Work out the finished part from the listing and answer in its coordinate system (mm). Round coordinates to 2 decimals unless told otherwise and drop trailing zeros. Write each loop counter-clockwise with the first axis right and the second up, starting at its lowest first coordinate (ties: lowest second). Pieces come first, ordered by that corner, then holes. Notation, with made-up numbers: (50.25, 76.5) -> (58.25, 76.5) arc R33 cw to (58.25, 108.5) -> close; hole circle Ø7 at (-17.75, 27.5). An arc over 180 degrees is marked (long way). One line per item, written item: value.
```python
from build123d import *

# Parameters (mm, degrees)
SZKIC1_R                    = 11
DODANIE_WYCI_GNI_CIE1_DEPTH = 5.25
ZAOKR_GLENIE1_R             = 0.2


with BuildPart() as part:
    # Szkic1 → Dodanie-wyciągnięcie1 (new body, symmetric)
    with BuildSketch(Plane(origin=(0, 0, 0), x_dir=(1, 0, 0), z_dir=(0, 1, 0))):
        Circle(SZKIC1_R)
    extrude(amount=DODANIE_WYCI_GNI_CIE1_DEPTH, both=True)

    # Szkic3 → Wycięcie-obrót1 (revolve, cut)
    with BuildSketch(Plane.XY):
        with BuildLine():
            Line((0, -9.52), (0, 9.52))
            ThreePointArc((0, 9.52), (9.52, 0), (0, -9.52))
        make_face()
    revolve(axis=Axis((0, -9.52, 0), (0, 1, 0)), mode=Mode.SUBTRACT)

    # Zaokrąglenie1
    zaokr_glenie1_edges = [part.edges().sort_by_distance(p)[0] for p in [
        (-11, -5.25, 0),
        (-11, 5.25, 0),
    ]]
    fillet(zaokr_glenie1_edges, radius=ZAOKR_GLENIE1_R)


solid = part.part
```
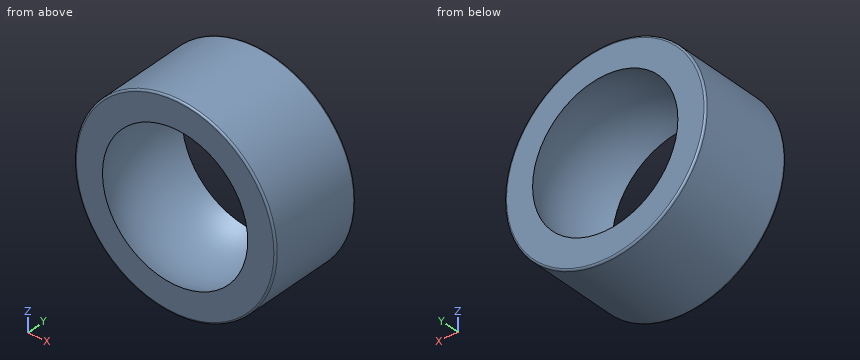
(1) Find section A-A on z = 0. Give the vertices of the cut face in (x, y), plus the area to 3 significant figures.
Reported:
outline: (-11, -5.05) arc R0.2 ccw to (-10.8, -5.25) -> (-7.94, -5.25) arc R9.52 cw to (-7.94, 5.25) -> (-10.8, 5.25) arc R0.2 ccw to (-11, 5.05) -> close; (7.94, -5.25) -> (10.8, -5.25) arc R0.2 ccw to (11, -5.05) -> (11, 5.05) arc R0.2 ccw to (10.8, 5.25) -> (7.94, 5.25) arc R9.52 cw to start
area: 41.7 mm2
(2) Find section D-D on y = -3.5. Give the vertices of the cut face in (x, z).
Reported:
outline: circle Ø22 at (0, 0); hole circle Ø17.71 at (0, 0)
(3) Flat-ended cylindrical pins translate along their axes: pin 1 Ø4 at (y, z) = (3.5, 4.5) entering from -X; pin 2 Ø4 at (y, z) = (-0.5, 4) entering from -X; pin 3 Ø6 at (x, y) = (-5, -3.5) entering from -Z. Find the tip coordinate at first contact, or state that the pin passes through.
Reported:
pin 1: stops at x = -10.71
pin 2: stops at x = -10.82
pin 3: stops at z = -10.82
(4) Consider probe 1 along X at (y, z) = (2.25, -1.75); probe 2 along Z at (x, y) = (0, 4.25); probe 3 along Z at (x, y) = (-2.75, 4.5). Determine where each line is inside the solid, lowest interval first.
Reported:
probe 1: x = -10.86 to -9.08, 9.08 to 10.86
probe 2: z = -11 to -8.52, 8.52 to 11
probe 3: z = -10.65 to -7.93, 7.93 to 10.65
(5) Find section B-B on x = 0. Give the vertices of the cut face in (y, z).
Reported:
outline: (-5.25, -10.8) arc R0.2 ccw to (-5.05, -11) -> (5.05, -11) arc R0.2 ccw to (5.25, -10.8) -> (5.25, -7.94) arc R9.52 cw to (-5.25, -7.94) -> close; (-5.25, 7.94) arc R9.52 cw to (5.25, 7.94) -> (5.25, 10.8) arc R0.2 ccw to (5.05, 11) -> (-5.05, 11) arc R0.2 ccw to (-5.25, 10.8) -> close
(6) Find section C-C on y = 1.5. Give the vertices of the cut face in (x, z).
Reported:
outline: circle Ø22 at (0, 0); hole circle Ø18.8 at (0, 0)
